Check sheet for the modelled part. Datum: model origin and axes. Units: mm. A direction names the side the tool comes from. Coordinates: 2 decimals unless noted, no trailing zeros. Write each loop counter-clockwise with the first axis right and the second up, starting at its lowest first coordinate (ties: lowest second). Pieces come first, ordered by that corner, then holes. Notation, with made-up numbers: M -2,30.5 L 17,30.5 A21 cw 17,59.5 Z; hole C 76.5,27.25 d1. An arc over 180 degrees is marked long. Answer as CSV lines item,"result". Start each with the question number.
Q1. Sectioned sample at A-A, the plane y = 0. Record the cut outline in (x, z), then the cut area to 3 significant figures.
Q2. Sectioned sample at D-D, the plane x = -1.25. Record the cut outline in (y, z), then the cut area to 3 significant figures.
Q3. Access from +Z, -Z, +X, -X, +Y, -Y to the whole of each face (thin tool, end or side, straight path). Record for faces 5 (the flat face through (-1, 4, 4.5)), 6 (the flat face through (-0.272, 4.377, -5.007)), 7 (the flat face through (4.4, 0.1, -4.25)), 8 (the cylindrical face through (-2.222, -10.006, 4.884)).
Q4. Thickness scan on line 1 along Y through (x, z) = (0, 3.25); line 2 along Z through (x, y) = (-5.5, -1.5); line 3 along X through (y, z) = (3.75, -5). Record the ranges inside material, lowest first. Write a range as from..to.
Q5. Sectioned sample at C-C, the plane z = -1.75. Record the cut outline in (x, y), then the cut area to 3 significant figures.
Q6. Depth check by flat-ended pin: pin 1 Ø2 at (y, z) = (8, 1.5) entering from +X; pin 2 Ø5 at (y, z) = (-4, 2.5) entering from -X; pin 3 Ø2 at (x, z) = (-7, 4) entering from +Y; pin 4 Ø2 at (x, z) = (3, 0.5) entering from -Y. Enter the tip coordinate at first touch or a pass-through.
Q7. Sectioned sample at B-B, the plane x = -4.5. Record the cut outline in (y, z), then the cut area to 3 significant figures.
Q8. Mould release check, pull along Y, two halves, no side actions. Record for faces 1 (the flat face through (-0.29, 4.34, 5.01)), 2 (the cylindrical face through (2.285, 3.584, -0.059)), 3 (the flat face through (-2.184, 3.787, -5.007)), 4 (the flat face through (0, -4, -5.5)): pulls with the +Y half, pulls with the -Y half, needs draft (parallel to the pull), parting line crosses it, or undercut.
from build123d import *

# Parameters (mm, degrees)
F0_R     = 10.25
F0_R_2   = 4.9
F0_R_3   = 3.4
F1_DEPTH = 5.5
F2_R     = 10.25
F2_R_2   = 4.25
F3_DEPTH = 4.25
F5_DEPTH = 1
F7_DEPTH = 1


with BuildPart() as f1:
    # F0 (on Top) → F1 (new body, symmetric)
    with BuildSketch(Plane.XY):
        Circle(F0_R)
        Circle(F0_R_2, mode=Mode.SUBTRACT)
        Circle(F0_R_2)
        Circle(F0_R_3, mode=Mode.SUBTRACT)
    extrude(amount=F1_DEPTH, both=True)

    # F2 (on Top) → F3 (cut, symmetric)
    with BuildSketch(Plane.XY):
        Circle(F2_R)
        Circle(F2_R_2, mode=Mode.SUBTRACT)
    extrude(amount=F3_DEPTH, both=True, mode=Mode.SUBTRACT)

    # F4 (on face) → F5 (cut)
    with BuildSketch(Plane.XY.offset(5.5)):
        with BuildLine():
            ThreePointArc((-1.911538, 2.811765), (-1, 3.249615), (0, 3.4))
            Line((0, 3.4), (-0.588235, 5.311538))
            Line((-0.588235, 5.311538), (-2.499774, 4.723303))
            Line((-2.499774, 4.723303), (-1.911538, 2.811765))
        make_face()
    extrude(amount=-F5_DEPTH, mode=Mode.SUBTRACT)

    # F6 (on face) → F7 (cut)
    with BuildSketch(Plane(origin=(0, 0, -5.5), x_dir=(1, 0, 0), z_dir=(0, 0, -1))):
        with BuildLine():
            ThreePointArc((0, -3.4), (-0.992761, -3.224814), (-1.912165, -2.811339))
            Line((-1.912165, -2.811339), (-2.463429, -4.789791))
            Line((-2.463429, -4.789791), (-0.536819, -5.32661))
            Line((-0.536819, -5.32661), (0, -3.4))
        make_face()
    extrude(amount=-F7_DEPTH, mode=Mode.SUBTRACT)


solid = f1.part
Output:
1,outline,"M -10.25,-5.5 L -3.4,-5.5 L -3.4,5.5 L -10.25,5.5 L -10.25,4.25 L -4.25,4.25 L -4.25,-4.25 L -10.25,-4.25 Z; M 3.4,-5.5 L 10.25,-5.5 L 10.25,-4.25 L 4.25,-4.25 L 4.25,4.25 L 10.25,4.25 L 10.25,5.5 L 3.4,5.5 Z"
1,area,"48.7 mm^2"
2,outline,"M -10.17,-5.5 L -3.16,-5.5 L -3.16,5.5 L -10.17,5.5 L -10.17,4.25 L -4.06,4.25 L -4.06,-4.25 L -10.17,-4.25 Z; M 3.16,-4.5 L 5.13,-4.5 L 5.13,-5.5 L 10.17,-5.5 L 10.17,-4.25 L 4.06,-4.25 L 4.06,4.25 L 10.17,4.25 L 10.17,5.5 L 5.11,5.5 L 5.11,4.5 L 3.16,4.5 Z"
2,area,"46.4 mm^2"
3,face 5,"+Z"
3,face 6,"-Z"
3,face 7,"none"
3,face 8,"+Z, -Z"
4,line 1,"y = -4.25..-3.4, 3.4..4.25"
4,line 2,"z = -5.5..-4.25, 4.25..5.5"
4,line 3,"x = -9.54..-2.17, -0.1..9.54"
5,outline,"C 0,0 d8.5; hole C 0,0 d6.8"
5,area,"20.4 mm^2"
6,pin 1,"passes through"
6,pin 2,"stops at x = -10.01"
6,pin 3,"stops at y = 8.29"
6,pin 4,"stops at y = -3.75"
7,outline,"M -9.21,-5.5 L 9.21,-5.5 L 9.21,-4.25 L -9.21,-4.25 Z; M -9.21,4.25 L 9.21,4.25 L 9.21,5.5 L -9.21,5.5 Z"
7,area,"46.0 mm^2"
8,face 1,"undercut"
8,face 2,"parting line crosses it"
8,face 3,"undercut"
8,face 4,"needs draft"
